The listing builds one solid part. Answer for the finished solid, in the listing's coordinates (mm). Round coordinates to 2 decimals unless told otherwise and drop trailing zeros. Write each loop counter-clockwise with the first axis right and the second up, starting at its lowest first coordinate (ties: lowest second). Pieces come first, ordered by that corner, then holes. Notation, with made-up numbers: (53, -13.75) - (84, -13.75) arc R13 ccw to (84, 2.25) - close; hole circle Ø10 at (18.5, 60). An arc over 180 degrees is marked (long way). Return JSON: item names as keys, results as strings. Group by question number.
(1) Section C-C, the plane y = -2.15 is taken. Write down the section's boundary in (x, z).
(2) Each of these flat-tipped pins is pushed along its axis until it touches: pin 1 (0.9 mm diameter, centred on y = -1.5, z = 8, fed in from -X); pin 2 (0.9 mm diameter, centred on y = -1.5, z = -9, fed in from +X); pin 3 (0.9 mm diameter, centred on y = -1, z = -8.5, fed in from +X). Where does it stop, or does it pass through?
(3) Find the intervals of material crossed by line 1 along Z through (x, y) = (-40, -1.65); line 2 along X through (y, z) = (-1.6, 4.5); line 3 along X through (y, z) = (-2.3, 8.5), in increasing order. Write a range as [from, to].
(4) Section A-A, the plane z = 0 is taken. Write down the section's boundary in (x, y).
(5) Section D-D, the plane z = -7.5 is taken. Write down the section's boundary in (x, y), then the cut area to 3 significant figures.
(6) Section B-B, the plane x = -17.5 is taken. Write down the section's boundary in (y, z), then the cut area to 3 significant figures.
```python
from build123d import *

# Parameters (mm, degrees)
F0_R     = 5
F0_R_2   = 2
F0_W     = 20
F0_H     = 4
F1_DEPTH = 3


with BuildPart() as f1:
    # F0 (on Front) → F1 (new body)
    with BuildSketch(Plane.XZ):
        with BuildLine():
            Line((-29, 10), (-40, 10))
            ThreePointArc((-40, 10), (-50, 0), (-40, -10))
            Line((-40, -10), (-29, -10))
            Line((-29, -10), (-29, -6))
            Line((-29, -6), (-25, -6))
            Line((-25, -6), (-25, -10))
            Line((-25, -10), (25, -10))
            Line((25, -10), (25, -6))
            Line((25, -6), (29, -6))
            Line((29, -6), (29, -10))
            Line((29, -10), (40, -10))
            ThreePointArc((40, -10), (50, 0), (40, 10))
            Line((40, 10), (29, 10))
            Line((29, 10), (29, 6))
            Line((29, 6), (25, 6))
            Line((25, 6), (25, 10))
            Line((25, 10), (-25, 10))
            Line((-25, 10), (-25, 6))
            Line((-25, 6), (-29, 6))
            Line((-29, 6), (-29, 10))
        make_face()
        with Locations((-40, 0)):
            Circle(F0_R, mode=Mode.SUBTRACT)
        with Locations((-17.5, 0)):
            Circle(F0_R_2, mode=Mode.SUBTRACT)
        Rectangle(F0_W, F0_H, mode=Mode.SUBTRACT)
        with Locations((17.5, 0)):
            Circle(F0_R_2, mode=Mode.SUBTRACT)
        with Locations((40, 0)):
            Circle(F0_R, mode=Mode.SUBTRACT)
    extrude(amount=F1_DEPTH)


solid = f1.part
```
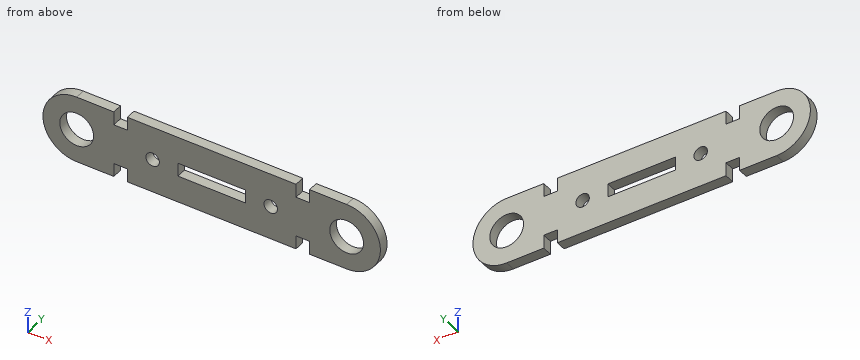
Working result:
{
 "1": {"outline": "(-40, -10) - (-29, -10) - (-29, -6) - (-25, -6) - (-25, -10) - (25, -10) - (25, -6) - (29, -6) - (29, -10) - (40, -10) arc R10 ccw to (40, 10) - (29, 10) - (29, 6) - (25, 6) - (25, 10) - (-25, 10) - (-25, 6) - (-29, 6) - (-29, 10) - (-40, 10) arc R10 ccw to start; hole circle Ø10 at (-40, 0); hole circle Ø4 at (-17.5, 0); hole (-10, -2) - (10, -2) - (10, 2) - (-10, 2) - close; hole circle Ø4 at (17.5, 0); hole circle Ø10 at (40, 0)"},
 "2": {"pin 1": "stops at x = -46.56", "pin 2": "stops at x = 45.19", "pin 3": "stops at x = 45.93"},
 "3": {"line 1": "z = [-10, -5], [5, 10]", "line 2": "x = [-48.93, -42.18], [-37.82, 37.82], [42.18, 48.93]", "line 3": "x = [-45.27, -29], [-25, 25], [29, 45.27]"},
 "4": {"outline": "(-50, -3) - (-45, -3) - (-45, 0) - (-50, 0) - close; (-35, -3) - (-19.5, -3) - (-19.5, 0) - (-35, 0) - close; (-15.5, -3) - (-10, -3) - (-10, 0) - (-15.5, 0) - close; (10, -3) - (15.5, -3) - (15.5, 0) - (10, 0) - close; (19.5, -3) - (35, -3) - (35, 0) - (19.5, 0) - close; (45, -3) - (50, -3) - (50, 0) - (45, 0) - close"},
 "5": {"outline": "(-46.61, -3) - (-29, -3) - (-29, 0) - (-46.61, 0) - close; (-25, -3) - (25, -3) - (25, 0) - (-25, 0) - close; (29, -3) - (46.61, -3) - (46.61, 0) - (29, 0) - close", "area": "256 mm^2"},
 "6": {"outline": "(-3, -10) - (0, -10) - (0, -2) - (-3, -2) - close; (-3, 2) - (0, 2) - (0, 10) - (-3, 10) - close", "area": "48.0 mm^2"}
}
